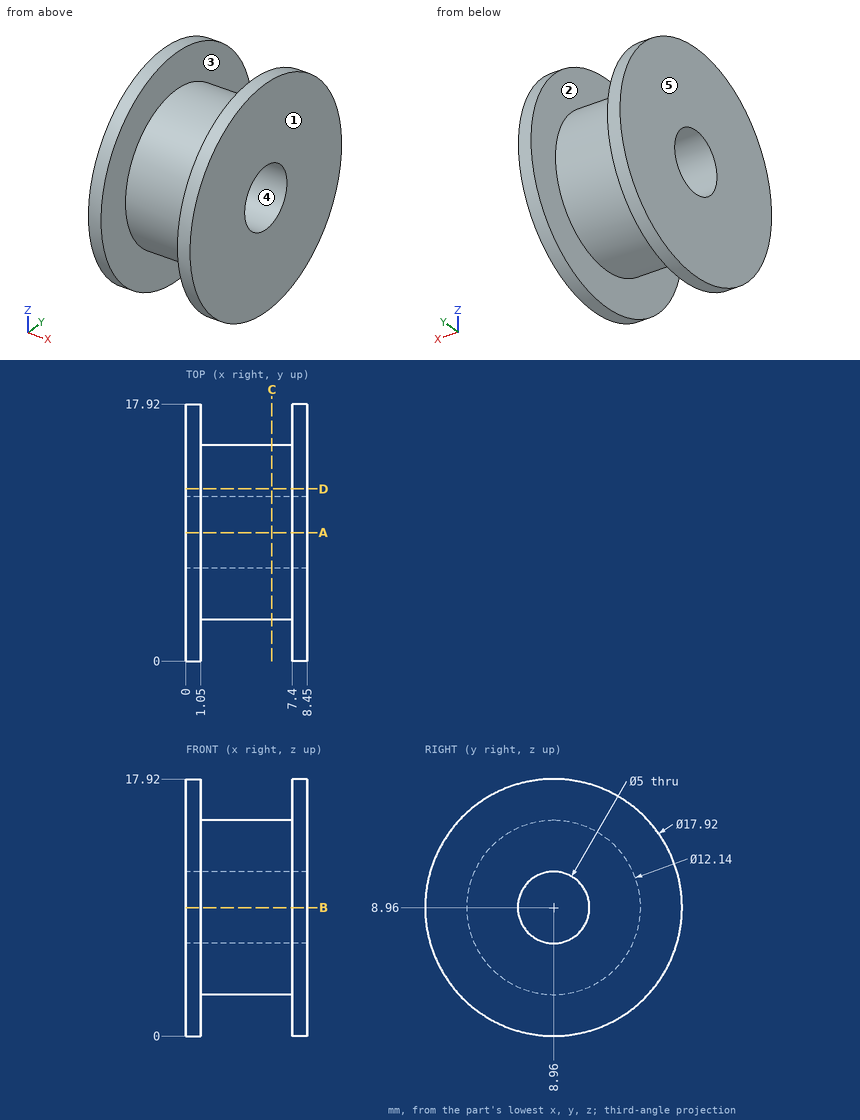
Job drawing, mm, ordinate dimensions from the low corner. One solid piece. A direction names the side the tool comes from. Give positions to 0.01 mm unless a question says otherwise; leave off trailing zeros. Loops run counter-clockwise (first coordinate to the right, second up) from the corner with the lowest first, then second, coordinate; pieces in that order, holes last. Notation, with made-up numbers: (60, 83) -> (79, 83) arc R36 cw to (79, 119) -> close; hole circle Ø5 at (32.25, 12). An arc over 180 degrees is marked (long way). Use a Markdown table: item, result. Add a question column.
(1) Slice it at D-D on y = 12. List the corners of the cut face in (x, z).
(2) Slice it at C-C on x = 6. List the corners of the cut face in (y, z), and give its area (3 significant figures).
(3) Slice it at A-A on y = 8.96. List the corners of the cut face in (x, z).
(4) Wall check: line 1 along Z through (x, y) = (6.75, 8.96); line 2 along X through (y, z) = (6.75, 1). Give the ranges that are in metal, low to high.
(5) Tool access for the marked faces 1 and 2: list every direction of +Z, -Z, +X, -X, +Y, -Y with a clear straight run to the whole face (end or side of a thin tool).
(6) Drop flat-ended pins along their axis: pin 1 Ø1 at (x, y) = (6.5, 2) entering from +Z; pin 2 Ø1 at (x, y) = (4, 6.5) entering from +Z. Give the stop position or say it passes through.
(7) Mould opens along X. For the marked faces 3, 4 and 5 say: +X half, -X half, draft (parallel to the pull), parting line (faces both ways), or undercut.
Filled sheet:
| question | item | result |
|---|---|---|
| 1 | outline | (0, 0.53) -> (1.05, 0.53) -> (1.05, 3.71) -> (7.4, 3.71) -> (7.4, 0.53) -> (8.45, 0.53) -> (8.45, 17.39) -> (7.4, 17.39) -> (7.4, 14.21) -> (1.05, 14.21) -> (1.05, 17.39) -> (0, 17.39) -> close |
| 2 | outline | circle Ø12.14 at (8.96, 8.96); hole circle Ø5 at (8.96, 8.96) |
| 2 | area | 96.1 mm2 |
| 3 | outline | (0, 0) -> (1.05, 0) -> (1.05, 2.89) -> (7.4, 2.89) -> (7.4, 0) -> (8.45, 0) -> (8.45, 6.46) -> (0, 6.46) -> close; (0, 11.46) -> (8.45, 11.46) -> (8.45, 17.92) -> (7.4, 17.92) -> (7.4, 15.03) -> (1.05, 15.03) -> (1.05, 17.92) -> (0, 17.92) -> close |
| 4 | line 1 | 2.89 to 6.46, 11.46 to 15.03 |
| 4 | line 2 | 0 to 1.05, 7.4 to 8.45 |
| 5 | face 1 | +Z, -Z, +X, +Y, -Y |
| 5 | face 2 | none |
| 6 | pin 1 | through |
| 6 | pin 2 | z = 14.7 |
| 7 | face 3 | undercut |
| 7 | face 4 | draft |
| 7 | face 5 | -X half |
